Autodesk Fusion 360 part; units mm, degrees
sketch "Sketch1" plane through (0, 0, 0) normal (0, 1, 0) x (1, 0, 0)
  line L0 (-65, 45) -> (65, 45)
  line L1 (65, 45) -> (65, -45)
  line L2 (65, -45) -> (-65, -45)
  line L3 (-65, -45) -> (-65, 45)
  circle A0 centre (55, 35.5) radius 1.65
  circle A1 centre (15, 35.5) radius 1.65
  circle A2 centre (55, -35.5) radius 1.65
  circle A3 centre (15, -35.5) radius 1.65
  dimension "d4" = 65
  dimension "d5" = 45
  dimension "d8" = 90
  dimension "d9" = 130
  dimension "d10" = 3.3
  dimension "d12" = 10
  dimension "d13" = 9.5
  dimension "d16" = -40
  dimension "d17" = -71
extrude "Extrude1" add sketch "Sketch1" along normal blind 7
sketch "Sketch2" plane through (0, 7, 0) normal (0, 1, 0) x (-1, 0, 0)
  circle A0 centre (-55, 35.5) radius 1.65
  circle A1 centre (-15, 35.5) radius 1.65
  circle A2 centre (-15, -35.5) radius 1.65
  circle A3 centre (-55, -35.5) radius 1.65
  line L0 (65, 45) -> (-65, 45)
  line L1 (-65, 45) -> (-65, -45)
  line L2 (-65, -45) -> (65, -45)
  line L3 (65, -45) -> (65, 45)
  line L4 (-45, -10) -> (20, -10)
  arc A4 (20, -10) -> (20, 10) centre (20, 0) ccw
  line L5 (20, 10) -> (-45, 10)
  arc A5 (-45, 10) -> (-45, -10) centre (-45, 0) ccw
  line L6 (-45, 0) -> (20, 0) construction
  dimension "d18" = 65
  dimension "d19" = 20
  dimension "d20" = 10
  dimension "d22" = 45
extrude "Extrude2" cut sketch "Sketch2" against normal up to surface (7 mm away) contours L4 A4 L5 A5
fillet "Fillet1" radius 5 4 edges at (65, 3.5, 45) (-65, 3.5, 45) (-65, 3.5, -45) (65, 3.5, -45)
sketch "Sketch3" plane through (0, 7, 0) normal (0, 1, 0) x (-1, 0, 0)
  arc A0 (-65, -40) -> (-60, -45) centre (-60, -40) ccw
  line L0 (-60, -45) -> (60, -45)
  arc A1 (60, -45) -> (65, -40) centre (60, -40) ccw
  line L1 (65, -40) -> (65, 40)
  arc A2 (65, 40) -> (60, 45) centre (60, 40) ccw
  line L2 (60, 45) -> (-60, 45)
  arc A3 (-60, 45) -> (-65, 40) centre (-60, 40) ccw
  line L3 (-65, 40) -> (-65, -40)
  line L4 (-45, 10) -> (20, 10)
  arc A4 (20, -10) -> (20, 10) centre (20, 0) ccw
  line L5 (20, -10) -> (-45, -10)
  arc A5 (-45, 10) -> (-45, -10) centre (-45, 0) ccw
  circle A6 centre (-55, 35.5) radius 1.65
  circle A7 centre (-15, 35.5) radius 1.65
  circle A8 centre (-15, -35.5) radius 1.65
  circle A9 centre (-55, -35.5) radius 1.65
  line L6 (57, -29.85) -> (15, -29.85)
  arc A10 (15, -29.85) -> (15, -33.15) centre (15, -31.5) ccw
  line L7 (15, -33.15) -> (57, -33.15)
  arc A11 (57, -33.15) -> (57, -29.85) centre (57, -31.5) ccw
  line L8 (57, -31.5) -> (15, -31.5) construction
  line L9 (0, 0) -> (102, 0) construction
  arc A12 (15, 33.15) -> (15, 29.85) centre (15, 31.5) ccw
  line L10 (15, 33.15) -> (57, 33.15)
  line L11 (57, 29.85) -> (15, 29.85)
  arc A13 (57, 29.85) -> (57, 33.15) centre (57, 31.5) ccw
  dimension "d26" = 3.3
  dimension "d27" = 8
  dimension "d28" = 42
  dimension "d30" = 31.5
extrude "Extrude3" cut sketch "Sketch3" against normal up to surface (7 mm away) contours L6 A10 L7 A11 | A12 L10 L11 A13
sketch "Sketch4" plane through (0, 0, 0) normal (0, -1, 0) x (1, 0, 0)
  line L0 (-15, -33.15) -> (-57, -33.15)
  arc A0 (-57, -29.85) -> (-57, -33.15) centre (-57, -31.5) ccw
  line L1 (-57, -29.85) -> (-15, -29.85)
  arc A1 (-15, -33.15) -> (-15, -29.85) centre (-15, -31.5) ccw
  line L2 (-57, 33.15) -> (-15, 33.15)
  arc A2 (-15, 29.85) -> (-15, 33.15) centre (-15, 31.5) ccw
  line L3 (-15, 29.85) -> (-57, 29.85)
  arc A3 (-57, 33.15) -> (-57, 29.85) centre (-57, 31.5) ccw
  line L4 (-20, 10) -> (45, 10)
  arc A4 (45, -10) -> (45, 10) centre (45, 0) ccw
  line L5 (45, -10) -> (-20, -10)
  arc A5 (-20, 10) -> (-20, -10) centre (-20, 0) ccw
  circle A6 centre (55, 35.5) radius 1.65
  circle A7 centre (15, 35.5) radius 1.65
  circle A8 centre (15, -35.5) radius 1.65
  circle A9 centre (55, -35.5) radius 1.65
  arc A10 (60, -45) -> (65, -40) centre (60, -40) ccw
  line L6 (65, -40) -> (65, 40)
  arc A11 (65, 40) -> (60, 45) centre (60, 40) ccw
  line L7 (60, 45) -> (-60, 45)
  arc A12 (-60, 45) -> (-65, 40) centre (-60, 40) ccw
  line L8 (-65, 40) -> (-65, -40)
  arc A13 (-65, -40) -> (-60, -45) centre (-60, -40) ccw
  line L9 (-60, -45) -> (60, -45)
  circle A14 centre (55, 35.5) radius 4
  circle A15 centre (55, -35.5) radius 4
  circle A16 centre (15, 35.5) radius 4
  circle A17 centre (15, -35.5) radius 4
  line L10 (-57, 27.5) -> (-15, 27.5)
  arc A18 (-15, 27.5) -> (-15, 35.5) centre (-15, 31.5) ccw
  line L11 (-15, 35.5) -> (-57, 35.5)
  arc A19 (-57, 35.5) -> (-57, 27.5) centre (-57, 31.5) ccw
  line L12 (-57, 31.5) -> (-15, 31.5) construction
  line L13 (-57, -35.5) -> (-15, -35.5)
  arc A20 (-15, -35.5) -> (-15, -27.5) centre (-15, -31.5) ccw
  line L14 (-15, -27.5) -> (-57, -27.5)
  arc A21 (-57, -27.5) -> (-57, -35.5) centre (-57, -31.5) ccw
  line L15 (-57, -31.5) -> (-15, -31.5) construction
  dimension "d33" = 8
  dimension "d34" = 8
  dimension "d35" = 8
  dimension "d36" = 8
  dimension "d37" = 8
  dimension "d38" = 8
extrude "Extrude4" cut sketch "Sketch4" against normal blind 3 contours A14 | A15 | A16 | A17 | L10 A18 L11 A19 | L13 A20 L14 A21
equation "length = 130 mm"
equation "width = 90 mm"
equation "thickness = 7 mm"
equation "d4 = length / 2"
equation "d5 = width / 2"
equation "d6 = thickness"
equation "d8 = width"
equation "d9 = length"
equation "d10 = d11"
equation "d13 = ( width - 71 mm ) / 2"
equation "d22 = width / 2"
equation "d30 = ( 63 / 2 ) * 1 mm"
Can you work these out from the model? Positions are in its coordinate system, mm. A direction names the side the tool comes from. Give positions to 0.01 mm unless a question says otherwise; leave off trailing zeros. Loops run counter-clockwise (first coordinate to the right, second up) from the corner with the lowest first, then second, coordinate; pieces in that order, holes last. Notation, with made-up numbers: (65.25, -11) - (83.25, -11) arc R14 cw to (83.25, 10) - close; hole circle Ø4 at (68.5, 85.5). An arc over 180 degrees is marked (long way). One line per item, written item: value.
(1) If we section it at D-D, the plane x = 48: List the corners of the cut face in (y, z) for me.
Verdict:
outline: (0, -45) - (7, -45) - (7, -9.54) - (0, -9.54) - close; (0, 9.54) - (7, 9.54) - (7, 45) - (0, 45) - close
(2) If we section it at A-A, the plane x = -34.5: List the corners of the cut face in (y, z) for me, plus the area to 3 significant figures.
Verdict:
outline: (0, -45) - (7, -45) - (7, -33.15) - (3, -33.15) - (3, -35.5) - (0, -35.5) - close; (0, -27.5) - (3, -27.5) - (3, -29.85) - (7, -29.85) - (7, 29.85) - (3, 29.85) - (3, 27.5) - (0, 27.5) - close; (0, 35.5) - (3, 35.5) - (3, 33.15) - (7, 33.15) - (7, 45) - (0, 45) - close
area: 556 mm^2
(3) If we mould it in two halves opening along X, with no side actions, what happens to faces 4 (the face through (-58.65, 5.03, -31.54)), 5 (the face through (-63, 4, -44)), 6 (the face through (-1, 7, -11))? For each: released by +X, released by -X, zero draft, split by the parting line, or undercut.
Verdict:
face 4: undercut
face 5: released by -X
face 6: zero draft
(4) On a 3-axis mill with a long thin cutter (end or side, diameter ignored), from which of +Z, -Z, +X, -X, +Y, -Y can I reach the whole of each face in a straight line? I mean faces 1 (the face through (12, 4, 10)), 2 (the face through (17, 3, 36)), 3 (the face through (1, 3, 45)). Say none if no direction works.
Verdict:
face 1: +Y, -Y
face 2: -Y
face 3: +Z, +X, -X, +Y, -Y
(5) If we section it at C-C, the plane z = 0: List the corners of the cut face in (x, y) for me, plus the area to 3 significant figures.
Verdict:
outline: (-65, 0) - (-30, 0) - (-30, 7) - (-65, 7) - close; (55, 0) - (65, 0) - (65, 7) - (55, 7) - close
area: 315 mm^2
(6) I need wall thicknesses on line 1 along X through (y, z) = (3.9, -35.5); line 2 along Z through (x, y) = (-42, 2.75); line 3 along Z through (x, y) = (-37, 4.5). Which ranges of each line are inside material? Lowest first, please.
Verdict:
line 1: -65 to 13.35, 16.65 to 53.35, 56.65 to 65
line 2: -45 to -35.5, -27.5 to 27.5, 35.5 to 45
line 3: -45 to -33.15, -29.85 to 29.85, 33.15 to 45
(7) I'm going to push a flat-ended pin straight in: pin 1 (7 mm diameter, centred on x = 15, z = 35.5, fed in from -Y). Where does the tip first touch, or does it pass through?
Verdict:
pin 1: y = 3
(8) If we section it at B-B, the plane x = 15: List the corners of the cut face in (y, z) for me.
Verdict:
outline: (0, -45) - (7, -45) - (7, -37.15) - (3, -37.15) - (3, -39.5) - (0, -39.5) - close; (0, -31.5) - (3, -31.5) - (3, -33.85) - (7, -33.85) - (7, -10) - (0, -10) - close; (0, 10) - (7, 10) - (7, 33.85) - (3, 33.85) - (3, 31.5) - (0, 31.5) - close; (0, 39.5) - (3, 39.5) - (3, 37.15) - (7, 37.15) - (7, 45) - (0, 45) - close
